```python
from build123d import *

# Parameters (mm, degrees)
CROQUIS1_W              = 45
CROQUIS1_H              = 45
CROQUIS1_W_2            = 6
CROQUIS1_H_2            = 3
SALIENTE_EXTRUIR1_DEPTH = 3
CROQUIS1_4_W            = 6
CROQUIS1_4_H            = 5
SALIENTE_EXTRUIR2_DEPTH = 3
CROQUIS2_R              = 10
CORTAR_EXTRUIR3_DEPTH   = 4
CROQUIS1_5_W            = 6
CROQUIS1_5_H            = 5
SALIENTE_EXTRUIR3_DEPTH = 3


with BuildPart() as part:
    # Croquis1 → Saliente-Extruir1 (new body)
    with BuildSketch(Plane(origin=(0, 0, 0), x_dir=(1, 0, 0), z_dir=(0, 1, 0))):
        Rectangle(CROQUIS1_W, CROQUIS1_H)
        with Locations((-14.5, 24)):
            Rectangle(CROQUIS1_W_2, CROQUIS1_H_2)
        with Locations((14.5, 24)):
            Rectangle(CROQUIS1_W_2, CROQUIS1_H_2)
        with Locations((14.5, -24)):
            Rectangle(CROQUIS1_W_2, CROQUIS1_H_2)
        with Locations((-14.5, -24)):
            Rectangle(CROQUIS1_W_2, CROQUIS1_H_2)
    extrude(amount=SALIENTE_EXTRUIR1_DEPTH)

    # Croquis1_4 → Saliente-Extruir2 (add)
    with BuildSketch(Plane(origin=(0, 0, 0), x_dir=(1, 0, 0), z_dir=(0, 1, 0))):
        with Locations((25.5, -10)):
            Rectangle(CROQUIS1_4_W, CROQUIS1_4_H)
        with Locations((-25.5, -10)):
            Rectangle(CROQUIS1_4_W, CROQUIS1_4_H)
    extrude(amount=SALIENTE_EXTRUIR2_DEPTH)

    # Croquis2 → Cortar-Extruir3 (cut, through all)
    with BuildSketch(Plane(origin=(0, 3, 0), x_dir=(1, 0, 0), z_dir=(0, 1, 0))):
        with Locations((-9.192388155, -9.192388155)):
            Circle(CROQUIS2_R)
        with Locations((9.192388155, 9.192388155)):
            Circle(CROQUIS2_R)
    extrude(amount=-CORTAR_EXTRUIR3_DEPTH, mode=Mode.SUBTRACT)

    # Croquis1_5 → Saliente-Extruir3 (add)
    with BuildSketch(Plane(origin=(0, 0, 0), x_dir=(1, 0, 0), z_dir=(0, 1, 0))):
        with Locations((-25.5, 10)):
            Rectangle(CROQUIS1_5_W, CROQUIS1_5_H)
        with Locations((25.5, 10)):
            Rectangle(CROQUIS1_5_W, CROQUIS1_5_H)
    extrude(amount=SALIENTE_EXTRUIR3_DEPTH)


solid = part.part
```
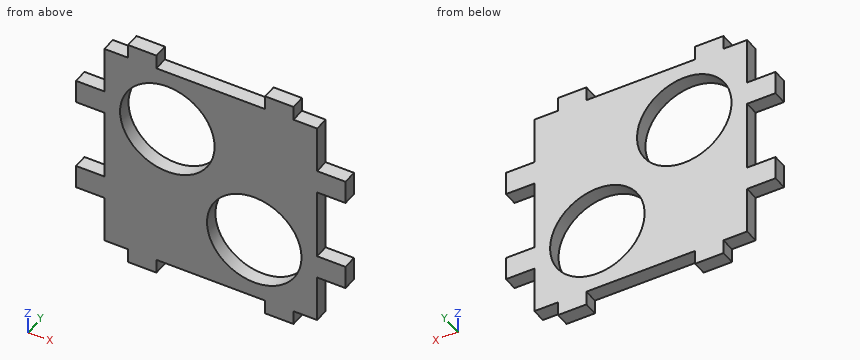
The listing builds one solid part. Answer for the finished solid, in the listing's coordinates (mm). Give positions to 0.01 mm unless a question says otherwise; leave off trailing zeros. Order: outer loops, then holes, each group sorted by start corner. A loop starts at its lowest first (then second) coordinate and runs counter-clockwise, first axis right, second up.
Item 1: The part is cut by section B-B, the plane z = -13.5. Give the vertices of the cut face in (x, y).
From the geometry:
outline: (-22.5, 0) - (0.17, 0) - (0.17, 3) - (-22.5, 3) - close; (18.22, 0) - (22.5, 0) - (22.5, 3) - (18.22, 3) - close
Item 2: Given pin 1 Ø0.9 at (y, z) = (1.5, -23.5) entering from +X; pin 2 Ø1.5 at (x, y) = (24, 1.5) entering from -Z; pin 3 Ø0.9 at (y, z) = (1.5, -24) entering from -X, each flat-ended and moving along its own axis, determine where each tip first touches the part or whether it passes through.
From the geometry:
pin 1: stops at x = 17.5
pin 2: stops at z = -12.5
pin 3: stops at x = -17.5
Item 3: The part is cut by section A-A, the plane x = -16. Give the vertices of the cut face in (y, z).
From the geometry:
outline: (0, -25.5) - (3, -25.5) - (3, 1.87) - (0, 1.87) - close; (0, 16.52) - (3, 16.52) - (3, 25.5) - (0, 25.5) - close
Item 4: The part is cut by section D-D, the plane y = 1.6. Count the separate pieces of the cut face and the enclosed holes in it, and give its area (3 significant figures).
From the geometry:
separate pieces: 1
enclosed holes: 2
area: 1,590 mm2
Item 5: Find the intervals of material crossed by probe 1 along Z at (x, y) = (23, 2.4); probe 2 along X at (y, z) = (1.5, 23); probe 3 along Z at (x, y) = (6, 2.75), in increasing order.
From the geometry:
probe 1: z = -12.5 to -7.5, 7.5 to 12.5
probe 2: x = -17.5 to -11.5, 11.5 to 17.5
probe 3: z = -22.5 to -18.67, 0.28 to 22.5
Item 6: The part is cut by section C-C, the plane x = 0. Give the vertices of the cut face in (y, z).
From the geometry:
outline: (0, -22.5) - (3, -22.5) - (3, -13.13) - (0, -13.13) - close; (0, -5.26) - (3, -5.26) - (3, 5.26) - (0, 5.26) - close; (0, 13.13) - (3, 13.13) - (3, 22.5) - (0, 22.5) - close
